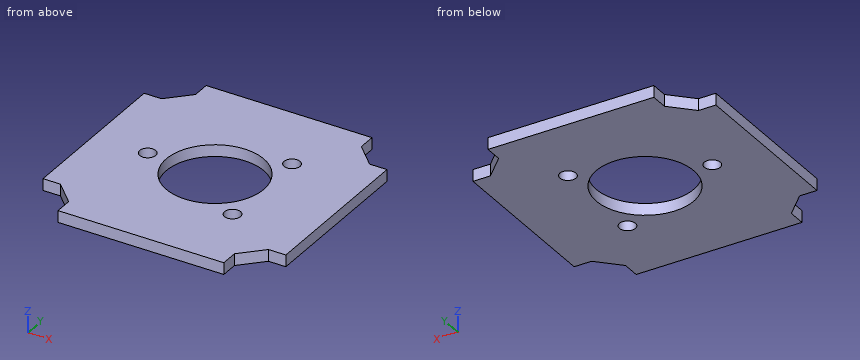
Autodesk Inventor part; units mm, degrees
ref_plane "Work Plane1" through (-29.1, -14.5, 2.4) normal (0, 0, -1) x (0, 1, 0)
ref_plane "YZ Plane" through (0, 0, 0) normal (1, 0, 0) x (0, 1, 0)
ref_plane "XZ Plane" through (0, 0, 0) normal (0, 1, 0) x (-1, 0, 0)
ref_plane "Work Plane1" through (-29.1, -14.5, 2.4) normal (0, 0, -1) x (0, 1, 0)
sketch "Sketch1" plane through (0, 0, 0) normal (0, 0, 1) x (1, 0, 0)
  line L0 (-34.86, 0) -> (34.86, 0) construction
  line L1 (0, -34.86) -> (0, 34.86) construction
  line L2 (0, 0) -> (11.1575, 11.1575) construction
  line L3 (0, 0) -> (15.7791, 0) construction
  line L4 (0, 24.9) -> (16.8009, 24.9)
  line L5 (16.8009, 24.9) -> (16.8009, 21.2415)
  line L6 (16.8009, 21.2415) -> (19.0212, 19.0212)
  line L7 (24.9, 0) -> (24.9, 16.8009)
  line L8 (24.9, 16.8009) -> (21.2415, 16.8009)
  line L9 (21.2415, 16.8009) -> (19.0212, 19.0212)
  line L10 (0, -24.9) -> (16.8009, -24.9)
  line L11 (16.8009, -24.9) -> (16.8009, -21.2415)
  line L12 (16.8009, -21.2415) -> (19.0212, -19.0212)
  line L13 (24.9, 0) -> (24.9, -16.8009)
  line L14 (24.9, -16.8009) -> (21.2415, -16.8009)
  line L15 (21.2415, -16.8009) -> (19.0212, -19.0212)
  line L16 (0, 24.9) -> (-16.8009, 24.9)
  line L17 (-16.8009, 24.9) -> (-16.8009, 21.2415)
  line L18 (-16.8009, 21.2415) -> (-19.0212, 19.0212)
  line L19 (-24.9, 16.8009) -> (-21.2415, 16.8009)
  line L20 (-21.2415, 16.8009) -> (-19.0212, 19.0212)
  line L21 (0, -24.9) -> (-16.8009, -24.9)
  line L22 (-16.8009, -24.9) -> (-16.8009, -21.2415)
  line L23 (-16.8009, -21.2415) -> (-19.0212, -19.0212)
  line L24 (-21.2415, -16.8009) -> (-19.0212, -19.0212)
  line L25 (-24.9, -16.8009) -> (-21.2415, -16.8009)
  line L26 (-24.9, 0) -> (-24.9, -16.8009)
  line L27 (-24.9, 0) -> (-24.9, 16.8009)
  circle A0 centre (0, 0) radius 10
  dimension "d0" = 45
  dimension "d2" = 24.9
  dimension "d3" = 3.14
  dimension "d4" = 26.9
  dimension "d5" = 20
extrude "Extrusion1" add sketch "Sketch1" along normal up to surface (2.4 mm away)
sketch "Sketch5" plane through (0, 0, 0) normal (0, 0, -1) x (-1, 0, 0)
  circle A0 centre (-9.7, 10) radius 1.4
  circle A1 centre (-9.7, -10) radius 1.4
  circle A2 centre (13.8, 0) radius 1.4
  point P0 (0, 0)
hole "Hole1" at (9.7, 10, 0) at (-13.8, 0, 0) at (9.7, -10, 0) direction (0, 0, 1) diameter 3.3 depth 12 tip angle 118
sketch "Skizze6" plane through (-16.8009, 24.9, 2.4) normal (0, 0, 1) x (1, 0, 0)
  circle A0 centre (3.0009, -24.9) radius 1.65 construction
  circle A1 centre (26.5009, -14.9) radius 1.65 construction
  circle A2 centre (26.5009, -34.9) radius 1.65 construction
  circle A3 centre (16.8009, -24.9) radius 10 construction
  line L0 (33.6017, -3.6585) -> (33.6017, 0)
  line L1 (33.6017, 0) -> (0, 0) construction
  line L2 (0, 0) -> (0, -3.6585)
  line L3 (0, -3.6585) -> (-4.4406, -8.0991)
  line L4 (-4.4406, -8.0991) -> (-8.0991, -8.0991)
  line L5 (-8.0991, -8.0991) -> (-8.0991, -41.7009) construction
  line L6 (-8.0991, -41.7009) -> (-4.4406, -41.7009)
  line L7 (-4.4406, -41.7009) -> (0, -46.1415)
  line L8 (0, -46.1415) -> (0, -49.8)
  line L9 (0, -49.8) -> (33.6017, -49.8) construction
  line L10 (33.6017, -49.8) -> (33.6017, -46.1415)
  line L11 (33.6017, -46.1415) -> (38.0423, -41.7009)
  line L12 (38.0423, -41.7009) -> (41.7009, -41.7009)
  line L13 (41.7009, -41.7009) -> (41.7009, -8.0991) construction
  line L14 (41.7009, -8.0991) -> (38.0423, -8.0991)
  line L15 (38.0423, -8.0991) -> (33.6017, -3.6585)
  line L16 (-0.2, 0.2) -> (33.8017, 0.2) construction
  line L17 (33.8017, 0.2) -> (33.8017, -3.5757)
  line L18 (33.8017, -3.5757) -> (38.1252, -7.8991)
  line L19 (38.1252, -7.8991) -> (41.9009, -7.8991)
  line L20 (41.9009, -7.8991) -> (41.9009, -41.9009) construction
  line L21 (41.9009, -41.9009) -> (38.1252, -41.9009)
  line L22 (38.1252, -41.9009) -> (33.8017, -46.2243)
  line L23 (33.8017, -46.2243) -> (33.8017, -50)
  line L24 (33.8017, -50) -> (-0.2, -50) construction
  line L25 (-0.2, -50) -> (-0.2, -46.2243)
  line L26 (-0.2, -46.2243) -> (-4.5235, -41.9009)
  line L27 (-4.5235, -41.9009) -> (-8.2991, -41.9009)
  line L28 (-8.2991, -41.9009) -> (-8.2991, -7.8991) construction
  line L29 (-8.2991, -7.8991) -> (-4.5235, -7.8991)
  line L30 (-4.5235, -7.8991) -> (-0.2, -3.5757)
  line L31 (-0.2, -3.5757) -> (-0.2, 0.2)
  line L32 (-8.0991, -8.0991) -> (-8.0991, -7.8991)
  line L33 (0, -3.6585) -> (0, 0)
  line L34 (0, 0) -> (-0.2, 0)
  line L35 (33.6017, 0) -> (33.6017, -3.6585)
  line L36 (33.6017, 0) -> (33.8017, 0)
  line L37 (41.7009, -8.0991) -> (41.7009, -7.8991)
  line L38 (41.7009, -41.7009) -> (41.7009, -8.0991)
  line L39 (41.7009, -41.7009) -> (41.7009, -41.9009)
  line L40 (33.6017, -49.8) -> (0, -49.8)
  line L41 (33.6017, -49.8) -> (33.8017, -49.8)
  line L42 (0, -49.8) -> (-0.2, -49.8)
  line L43 (-8.0991, -41.7009) -> (-8.0991, -41.9009)
  dimension "d25" = 0.2
extrude "IM_offset" add sketch "Skizze6" against normal up to surface (2.4 mm away)
properties part number "20_Cube_insert_Basler_acA1920_25gm_v3"
Input: part model. Units: mm. Frame: model coordinates. Round coordinates to 2 decimals unless told otherwise and drop trailing zeros. Loops run counter-clockwise (first coordinate to the right, second up) from the corner with the lowest first, then second, coordinate; pieces in that order, holes last. Notation, with made-up numbers: (32, 9.25) -> (43, 9.25) arc R29 ccw to (43, 31.25) -> close; hole circle Ø7 at (35, 6.5). An arc over 180 degrees is marked (long way). One line per item, written item: value.
(1) Pin query (flat end, axial travel): pin 1 (6 mm diameter, centred on x = -10.5, y = 1.5, fed in from -Z); pin 2 (1.2 mm diameter, centred on x = 22.5, z = 1.5, fed in from -Y); pin 3 (0.7 mm diameter, centred on y = -23.5, z = 1.5, fed in from +X); pin 4 (0.7 mm diameter, centred on y = 22.5, z = 1, fed in from -X). Return the tip coordinate at first contact, or that it passes through.
Geometry check:
pin 1: z = 0
pin 2: y = -17
pin 3: x = 17
pin 4: x = -17
(2) Section C-C (y = -5.5). Return the cut outline in (x, z), plus the area to 3 significant figures.
Geometry check:
outline: (-24.9, 0) -> (-8.35, 0) -> (-8.35, 2.4) -> (-24.9, 2.4) -> close; (8.35, 0) -> (24.9, 0) -> (24.9, 2.4) -> (8.35, 2.4) -> close
area: 79.4 mm2
(3) Section A-A (x = -13.8). Return the cut outline in (y, z), plus the area to 3 significant figures.
Geometry check:
outline: (-24.9, 0) -> (-1.65, 0) -> (-1.65, 2.4) -> (-24.9, 2.4) -> close; (1.65, 0) -> (24.9, 0) -> (24.9, 2.4) -> (1.65, 2.4) -> close
area: 112 mm2
(4) Material intervals for line 1 (Y direction, x = -6.5, z = 1.5); line 2 (Y direction, x = 8.5, z = 0.45); line 3 (Y direction, x = -4, z = 2.15), sorted ascending. Write a range as [from, to].
Geometry check:
line 1: [-24.9, -7.6], [7.6, 24.9]
line 2: [-24.9, -11.13], [-8.87, -5.27], [5.27, 8.87], [11.13, 24.9]
line 3: [-24.9, -9.17], [9.17, 24.9]
(5) Section B-B (z = 0.5). Return the cut outline in (x, y), plus the area to 3 significant figures.
Geometry check:
outline: (-24.9, -17) -> (-21.32, -17) -> (-17, -21.32) -> (-17, -24.9) -> (17, -24.9) -> (17, -21.32) -> (21.32, -17) -> (24.9, -17) -> (24.9, 17) -> (21.32, 17) -> (17, 21.32) -> (17, 24.9) -> (-17, 24.9) -> (-17, 21.32) -> (-21.32, 17) -> (-24.9, 17) -> close; hole circle Ø3.3 at (-13.8, 0); hole circle Ø20 at (0, 0); hole circle Ø3.3 at (9.7, -10); hole circle Ø3.3 at (9.7, 10)
area: 1,930 mm2
(6) Section D-D (x = -20.5). Return the cut outline in (y, z), plus the area to 3 significant figures.
Geometry check:
outline: (-17.83, 0) -> (17.83, 0) -> (17.83, 2.4) -> (-17.83, 2.4) -> close
area: 85.6 mm2
